Geometry: final body of the model. Coordinates: model frame, mm. A direction names the side the tool comes from. Coordinates: 2 decimals unless noted, no trailing zeros. Loops run counter-clockwise (first coordinate to the right, second up) from the corner with the lowest first, then second, coordinate; pieces in that order, holes last. Notation, with made-up numbers: (9.5, 26) -> (56.5, 26) arc R11 cw to (56.5, 39) -> close; hole circle Ø6 at (89.5, 56). An arc over 180 degrees is marked (long way). One line per item, written item: value. Start each with the question number.
Item 1: Contact query for flat-ended pins moving along their axis: pin 1 Ø1 at (y, z) = (-1, 3) entering from +X; pin 2 Ø1.5 at (y, z) = (-8, 8.5) entering from -X; pin 3 Ø0.6 at (x, z) = (-5.5, 1) entering from +Y. Output: stop coordinate, or through.
Item 2: Ray query, probe 1 along Z at (x, y) = (-4, 3); probe 2 along Z at (x, y) = (16.5, -7); probe 3 along X at (y, z) = (-15, 3.75). Return the intervals inside material, ascending. Write a range as from..to.
Item 3: Section query A-A on z = 7.25. Return loops of the section in (x, y), then the cut area to 3 significant figures.
Item 4: Set-up query: faces 1 (the flat face through (1, -3, 0)), 2 (the flat face through (-10.223, 5, 1)). Return all of +Z, -Z, +X, -X, +Y, -Y with unobstructed straight access to the full face (end or side cutting, diameter ignored); none if empty.
from build123d import *

# Parameters (mm, degrees)
F0_R     = 21
F1_DEPTH = 5
F2_R     = 18.332
F3_DEPTH = 5
F4_R     = 0.831881
F5_DEPTH = 2
F6_SIZE  = 4


with BuildPart() as f1:
    # F0 (on Top) → F1 (new body)
    with BuildSketch(Plane.XY):
        Circle(F0_R)
    extrude(amount=F1_DEPTH)

    # F2 (on face) → F3 (join)
    with BuildSketch(Plane.XY.offset(5)):
        Circle(F2_R)
    extrude(amount=F3_DEPTH)

    # F4 (on face) → F5 (cut)
    with BuildSketch(Plane(origin=(0, 0, 0), x_dir=(1, 0, 0), z_dir=(0, 0, -1))):
        with BuildLine():
            Line((-8.597011, 1.060302), (-5.727476, 1.060302))
            ThreePointArc((-5.727476, 1.060302), (-4.950709, 3.036583), (-3.504453, 4.59138))
            Line((-3.504453, 4.59138), (-8.52302, 4.59138))
            ThreePointArc((-8.52302, 4.59138), (-9.17742, 4.328519), (-9.468151, 3.686015))
            ThreePointArc((-9.468151, 3.686015), (-10.070724, 3.645277), (-10.475405, 3.196962))
            Line((-10.475405, 3.196962), (-10.475405, 2.261244))
            ThreePointArc((-10.475405, 2.261244), (-10.072278, 1.81049), (-9.47128, 1.743463))
            ThreePointArc((-9.47128, 1.743463), (-9.151775, 1.251347), (-8.597011, 1.060302))
        make_face()
        with BuildLine():
            ThreePointArc((-3.504453, 4.59138), (-4.950709, 3.036583), (-5.727476, 1.060302))
            ThreePointArc((-5.727476, 1.060302), (-5.826342, 0.084509), (-5.756453, -0.893787))
            ThreePointArc((-5.756453, -0.893787), (-5.359136, -2.261429), (-4.635161, -3.487874))
            ThreePointArc((-4.635161, -3.487874), (1.715573, -5.393429), (5.572241, 0))
            ThreePointArc((5.572241, 0), (5.5686, 0.2037), (5.557681, 0.407141))
            ThreePointArc((5.557681, 0.407141), (4.75085, 2.947629), (2.877083, 4.843428))
            ThreePointArc((2.877083, 4.843428), (-0.352303, 5.695164), (-3.504453, 4.59138))
        make_face()
        with BuildLine():
            Line((-0.40257, -1.372951), (-0.40257, -4.237055))
            ThreePointArc((-0.40257, -4.237055), (-2.31047, -3.76336), (-3.696814, -2.369617))
            Line((-3.696814, -2.369617), (-1.0845, -0.953302))
            Line((-1.0845, -0.953302), (-0.40257, -1.372951))
        make_face(mode=Mode.SUBTRACT)
        with BuildLine():
            Line((0.216412, -4.289511), (0.216412, -1.488355))
            Line((0.216412, -1.488355), (0.961289, -0.953302))
            Line((0.961289, -0.953302), (3.426726, -2.526986))
            ThreePointArc((3.426726, -2.526986), (2.055218, -3.833824), (0.216412, -4.289511))
        make_face(mode=Mode.SUBTRACT)
        with BuildLine():
            Line((-1.556605, 0.546942), (-1.556605, -0.313338))
            Line((-1.556605, -0.313338), (-4.043024, -1.782109))
            ThreePointArc((-4.043024, -1.782109), (-4.506304, 0.234199), (-3.843691, 2.194064))
            Line((-3.843691, 2.194064), (-1.556605, 0.546942))
        make_face(mode=Mode.SUBTRACT)
        with Locations((-0.127364, 0)):
            Circle(F4_R, mode=Mode.SUBTRACT)
        with BuildLine():
            Line((-0.439486, 1.44269), (-1.070051, 1.197883))
            Line((-1.070051, 1.197883), (-3.436526, 2.770586))
            ThreePointArc((-3.436526, 2.770586), (-2.151244, 3.990055), (-0.439486, 4.447148))
            Line((-0.439486, 4.447148), (-0.439486, 1.44269))
        make_face(mode=Mode.SUBTRACT)
        with BuildLine():
            Line((3.821978, -1.8935), (1.325343, -0.287891))
            Line((1.325343, -0.287891), (1.325343, 0.506092))
            Line((1.325343, 0.506092), (3.689648, 1.997015))
            ThreePointArc((3.689648, 1.997015), (4.334116, 0.071428), (3.821978, -1.8935))
        make_face(mode=Mode.SUBTRACT)
        with BuildLine():
            Line((3.368104, 2.591078), (0.929, 1.075215))
            Line((0.929, 1.075215), (0.192902, 1.461979))
            Line((0.192902, 1.461979), (0.192902, 4.479774))
            ThreePointArc((0.192902, 4.479774), (2.033345, 3.960494), (3.368104, 2.591078))
        make_face(mode=Mode.SUBTRACT)
        with BuildLine():
            ThreePointArc((-4.635161, -3.487874), (-5.359136, -2.261429), (-5.756453, -0.893787))
            ThreePointArc((-5.756453, -0.893787), (-7.938026, -2.56399), (-10.222816, -4.089958))
            Line((-10.222816, -4.089958), (-10.222816, -5.373343))
            ThreePointArc((-10.222816, -5.373343), (-7.297319, -4.820816), (-4.635161, -3.487874))
        make_face()
        with BuildLine():
            Line((14.553333, 4.843428), (2.877083, 4.843428))
            ThreePointArc((2.877083, 4.843428), (4.75085, 2.947629), (5.557681, 0.407141))
            ThreePointArc((5.557681, 0.407141), (7.075636, 0.742717), (8.332674, 1.657405))
            Line((8.332674, 1.657405), (12.917255, 1.879957))
            Line((12.917255, 1.879957), (12.9363, 1.48763))
            Line((12.9363, 1.48763), (13.997183, 1.539129))
            ThreePointArc((13.997183, 1.539129), (14.516183, 3.150728), (14.553333, 4.843428))
        make_face()
    extrude(amount=-F5_DEPTH, mode=Mode.SUBTRACT)

    # F6
    f6_edges = [f1.edges().sort_by_distance(p)[0] for p in [
        (-21, 0, 0),
    ]]
    chamfer(f6_edges, length=F6_SIZE)


solid = f1.part
Reply:
1. pin 1: stops at x = 20.48
1. pin 2: stops at x = -16.84
1. pin 3: stops at y = 17.47
2. probe 1: z = 2..10
2. probe 2: z = 0.92..10
2. probe 3: x = -14.34..14.34
3. outline: circle Ø36.66 at (0, 0)
3. area: 1,060 mm²
4. face 1: -Z, +X, -X, +Y, -Y
4. face 2: -Z
